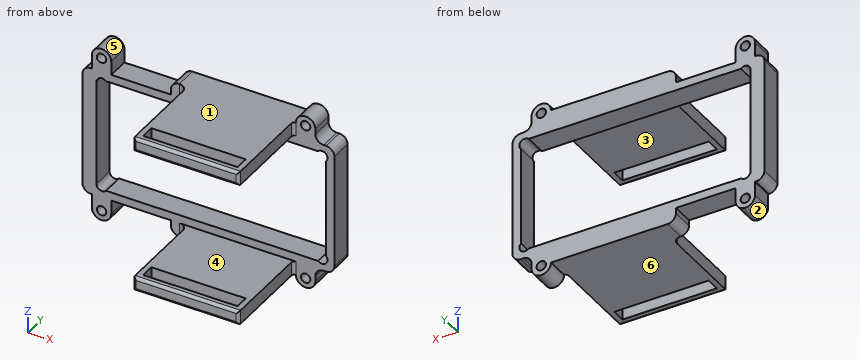
from build123d import *

# Parameters (mm, degrees)
EXTRUDE_1_DEPTH     = 23.5
EXTRUDE_START       = 8
SKETCH_2_R          = 1.7
EXTRUDE_2_DEPTH     = 8
CUT_EXTRUDE_1_REACH = 98.655
CUT_EXTRUDE_2_REACH = 79.127
CUT_EXTRUDE_3_REACH = 93.669
SKETCH_9_W          = 45
SKETCH_9_H          = 8
EXTRUDE_3_DEPTH     = 5
SKETCH_10_W         = 45
SKETCH_10_H         = 8
EXTRUDE_4_DEPTH     = 5
SKETCH_11_W         = 38
SKETCH_11_H         = 5
EXTRUDE_5_DEPTH     = 33
SKETCH_12_W         = 34
SKETCH_12_H         = 5
CUT_EXTRUDE_4_DEPTH = 5
CUT_EXTRUDE_START   = -23.5
CUT_EXTRUDE_5_DEPTH = 23.5
CUT_EXTRUDE_6_DEPTH = 67.550849919
FILLET_1_R          = 3
FILLET_2_R          = 1
FILLET_3_R          = 1


with BuildPart() as part:
    # 草图1 → 凸台-拉伸1 (new body)
    with BuildSketch(Plane(origin=(0, 0, 0), x_dir=(1, 0, 0), z_dir=(0, 1, 0))):
        with BuildLine():
            Line((-38, 23.5), (40, 23.5))
            Line((40, 23.5), (40, -23.5))
            Line((40, -23.5), (-38, -23.5))
            ThreePointArc((-38, -23.5), (-39.414213562, -22.914213562), (-40, -21.5))
            Line((-40, -21.5), (-40, 21.5))
            ThreePointArc((-40, 21.5), (-39.414213562, 22.914213562), (-38, 23.5))
        make_face()
        with BuildLine():
            Line((-34.171572875, -20.5), (36, -20.5))
            ThreePointArc((36, -20.5), (37.414213562, -19.914213562), (38, -18.5))
            Line((38, -18.5), (38, 18.5))
            ThreePointArc((38, 18.5), (37.414213562, 19.914213562), (36, 20.5))
            Line((36, 20.5), (-34.171572875, 20.5))
            ThreePointArc((-34.171572875, 20.5), (-37, 20.5), (-37, 17.671572875))
            Line((-37, 17.671572875), (-37, -17.671572875))
            ThreePointArc((-37, -17.671572875), (-37, -20.5), (-34.171572875, -20.5))
        make_face(mode=Mode.SUBTRACT)
    extrude(amount=EXTRUDE_1_DEPTH)

    # 草图2 → 凸台-拉伸2 (add)
    with BuildSketch(Plane.XZ.offset(EXTRUDE_START)):
        with BuildLine():
            Line((48.125, 23.5), (41.25, 23.5))
            Line((41.25, 23.5), (41.25, 28.5))
            ThreePointArc((41.25, 28.5), (37.75, 32), (34.25, 28.5))
            Line((34.25, 28.5), (34.25, 23.5))
            Line((34.25, 23.5), (-32.25, 23.5))
            Line((-32.25, 23.5), (-32.25, 28.5))
            ThreePointArc((-32.25, 28.5), (-35.75, 32), (-39.25, 28.5))
            Line((-39.25, 28.5), (-39.25, 23.5))
            Line((-39.25, 23.5), (-42.625, 23.5))
            Line((-42.625, 23.5), (-42.625, -23.5))
            Line((-42.625, -23.5), (-39.25, -23.5))
            Line((-39.25, -23.5), (-39.25, -28.5))
            ThreePointArc((-39.25, -28.5), (-35.75, -32), (-32.25, -28.5))
            Line((-32.25, -28.5), (-32.25, -23.5))
            Line((-32.25, -23.5), (34.25, -23.5))
            Line((34.25, -23.5), (34.25, -28.5))
            ThreePointArc((34.25, -28.5), (37.75, -32), (41.25, -28.5))
            Line((41.25, -28.5), (41.25, -23.5))
            Line((41.25, -23.5), (48.125, -23.5))
            Line((48.125, -23.5), (48.125, 23.5))
        make_face()
        with Locations(Location((37.75, 28.5, 0), (0, 0, 270))):
            Circle(SKETCH_2_R, mode=Mode.SUBTRACT)
        with Locations(Location((37.75, -28.5, 0), (0, 0, 90))):
            Circle(SKETCH_2_R, mode=Mode.SUBTRACT)
        with Locations(Location((-35.75, -28.5, 0), (0, 0, 270))):
            Circle(SKETCH_2_R, mode=Mode.SUBTRACT)
        with Locations(Location((-35.75, 28.5, 0), (0, 0, 90))):
            Circle(SKETCH_2_R, mode=Mode.SUBTRACT)
        with BuildLine():
            Line((-34.171572875, 20.5), (42.231907087, 20.5))
            ThreePointArc((42.231907087, 20.5), (45.060334211, 20.5), (45.060334211, 17.671572875))
            Line((45.060334211, 17.671572875), (45.060334211, -17.671572875))
            ThreePointArc((45.060334211, -17.671572875), (45.060334211, -20.5), (42.231907087, -20.5))
            Line((42.231907087, -20.5), (-34.171572875, -20.5))
            ThreePointArc((-34.171572875, -20.5), (-37, -20.5), (-37, -17.671572875))
            Line((-37, -17.671572875), (-37, 17.671572875))
            ThreePointArc((-37, 17.671572875), (-37, 20.5), (-34.171572875, 20.5))
        make_face(mode=Mode.SUBTRACT)
    extrude(amount=-EXTRUDE_2_DEPTH)

    # 草图4 → 切除-拉伸1 (cut, up to next)
    with BuildSketch(Plane.ZY.offset(40), mode=Mode.PRIVATE) as cut_extrude_1_sk1:
        with BuildLine():
            Line((17, 0), (-17, 0))
            ThreePointArc((-17, 0), (-19.121320344, 0.878679656), (-20, 3))
            Line((-20, 3), (-20, 17.5))
            ThreePointArc((-20, 17.5), (-19.121320344, 19.621320344), (-17, 20.5))
            Line((-17, 20.5), (17, 20.5))
            ThreePointArc((17, 20.5), (19.121320344, 19.621320344), (20, 17.5))
            Line((20, 17.5), (20, 3))
            ThreePointArc((20, 3), (19.121320344, 0.878679656), (17, 0))
        make_face()
    cut_extrude_1_tool1 = extrude(cut_extrude_1_sk1.sketch, amount=-CUT_EXTRUDE_1_REACH, mode=Mode.PRIVATE) & part.part
    add(cut_extrude_1_tool1.solids().sort_by_distance((-40, 10.25, 0))[0], mode=Mode.SUBTRACT)

    # 切除-拉伸2: up to this face of the body (flat: up to its plane)
    cut_extrude_2_end = Plane(part.part.faces().sort_by_distance((1, 8.207082452, 23.5))[0])
    # 草图5 → 切除-拉伸2 (cut, up to the picked face)
    with BuildSketch(Plane(origin=(0, 0, -23.5), x_dir=(-1, 0, 0), z_dir=(0, 0, -1)), mode=Mode.PRIVATE) as cut_extrude_2_sk1:
        with BuildLine():
            Line((-37, 11.75), (-37, 17.5))
            ThreePointArc((-37, 17.5), (-36.414213562, 18.914213562), (-35, 19.5))
            Line((-35, 19.5), (33, 19.5))
            ThreePointArc((33, 19.5), (34.414213562, 18.914213562), (35, 17.5))
            Line((35, 17.5), (35, 6))
            ThreePointArc((35, 6), (34.414213562, 4.585786438), (33, 4))
            Line((33, 4), (-35, 4))
            ThreePointArc((-35, 4), (-36.414213562, 4.585786438), (-37, 6))
            Line((-37, 6), (-37, 11.75))
        make_face()
    cut_extrude_2_tool1 = split(extrude(cut_extrude_2_sk1.sketch, amount=-CUT_EXTRUDE_2_REACH, mode=Mode.PRIVATE), bisect_by=cut_extrude_2_end, keep=Keep.BOTH, mode=Mode.PRIVATE)
    add(cut_extrude_2_tool1.solids().sort_by(Axis((1, 11.75, -23.5), (0, 0, 1)))[0], mode=Mode.SUBTRACT)

    # 草图6 → 切除-拉伸3 (cut, up to next)
    with BuildSketch(Plane(origin=(40, 0, 0), x_dir=(0, 0, -1), z_dir=(1, 0, 0)), mode=Mode.PRIVATE) as cut_extrude_3_sk1:
        with BuildLine():
            Line((21, 5), (21, 18.5))
            ThreePointArc((21, 18.5), (20.414213562, 19.914213562), (19, 20.5))
            Line((19, 20.5), (-19, 20.5))
            ThreePointArc((-19, 20.5), (-20.414213562, 19.914213562), (-21, 18.5))
            Line((-21, 18.5), (-21, 5))
            Line((-21, 5), (-21, 0))
            Line((-21, 0), (-16, 0))
            Line((-16, 0), (16, 0))
            Line((16, 0), (21, 0))
            Line((21, 0), (21, 5))
        make_face()
    cut_extrude_3_tool1 = extrude(cut_extrude_3_sk1.sketch, amount=-CUT_EXTRUDE_3_REACH, mode=Mode.PRIVATE) & part.part
    add(cut_extrude_3_tool1.solids().sort_by_distance((40, 10.230413, 0))[0], mode=Mode.SUBTRACT)

    # 草图9 → 凸台-拉伸3 (add)
    with BuildSketch(Plane.XY.offset(23.5)):
        with Locations((11.75, -4)):
            Rectangle(SKETCH_9_W, SKETCH_9_H)
    extrude(amount=EXTRUDE_3_DEPTH)

    # 草图10 → 凸台-拉伸4 (add)
    with BuildSketch(Plane(origin=(0, 0, -23.5), x_dir=(-1, 0, 0), z_dir=(0, 0, -1))):
        with Locations((-11.75, -4)):
            Rectangle(SKETCH_10_W, SKETCH_10_H)
    extrude(amount=EXTRUDE_4_DEPTH)

    # 草图11 → 凸台-拉伸5 (add)
    with BuildSketch(Plane.XZ.offset(8)):
        with Locations((14.25, 26)):
            Rectangle(SKETCH_11_W, SKETCH_11_H)
    extrude_5 = extrude(amount=EXTRUDE_5_DEPTH)

    # 草图12 → 切除-拉伸4 (cut)
    with BuildSketch(Plane(origin=(0, 0, 23.5), x_dir=(-1, 0, 0), z_dir=(0, 0, -1))):
        with Locations((-14.25, -36)):
            Rectangle(SKETCH_12_W, SKETCH_12_H)
    cut_extrude_4 = extrude(amount=-CUT_EXTRUDE_4_DEPTH, mode=Mode.SUBTRACT)

    # 镜向1: 凸台-拉伸5, 切除-拉伸4 across plane
    add(extrude_5.mirror(Plane.XY))
    add(cut_extrude_4.mirror(Plane.XY), mode=Mode.SUBTRACT)

    # 草图13 → 切除-拉伸5 (cut)
    with BuildSketch(Plane(origin=(0, 23.5, 0), x_dir=(1, 0, 0), z_dir=(0, 1, 0)).offset(CUT_EXTRUDE_START)):
        with BuildLine():
            Line((-38, 23.5), (40, 23.5))
            Line((40, 23.5), (40, -23.5))
            Line((40, -23.5), (-38, -23.5))
            ThreePointArc((-38, -23.5), (-39.414213562, -22.914213562), (-40, -21.5))
            Line((-40, -21.5), (-40, 21.5))
            ThreePointArc((-40, 21.5), (-39.414213562, 22.914213562), (-38, 23.5))
        make_face()
        with BuildLine():
            Line((38, 18.5), (38, -18.5))
            ThreePointArc((38, -18.5), (37.414213562, -19.914213562), (36, -20.5))
            Line((36, -20.5), (-34.171572875, -20.5))
            ThreePointArc((-34.171572875, -20.5), (-37, -20.5), (-37, -17.671572875))
            Line((-37, -17.671572875), (-37, 17.671572875))
            ThreePointArc((-37, 17.671572875), (-37, 20.5), (-34.171572875, 20.5))
            Line((-34.171572875, 20.5), (36, 20.5))
            ThreePointArc((36, 20.5), (37.414213562, 19.914213562), (38, 18.5))
        make_face(mode=Mode.SUBTRACT)
    extrude(amount=CUT_EXTRUDE_5_DEPTH, mode=Mode.SUBTRACT)

    # 草图14 → 切除-拉伸6 (cut, through all)
    with BuildSketch(Plane.XZ.offset(8)):
        with BuildLine():
            Line((-37.585786438, 19.085786438), (-37.585786438, -19.085786438))
            ThreePointArc((-37.585786438, -19.085786438), (-37.433545503, -18.320419573), (-37, -17.671572875))
            Line((-37, -17.671572875), (-37, 17.671572875))
            ThreePointArc((-37, 17.671572875), (-37.433545503, 18.320419573), (-37.585786438, 19.085786438))
        make_face()
    extrude(amount=-CUT_EXTRUDE_6_DEPTH, mode=Mode.SUBTRACT)

    # 圆角1
    fillet_1_edges = [part.edges().sort_by_distance(p)[0] for p in [
        (-10.75, -4, 28.5),
        (-10.75, -4, -28.5),
        (-42.625, -4, 23.5),
        (-42.625, -4, -23.5),
        (-4.75, -8, 26),
        (-4.75, -8, -26),
        (41.25, -4, 23.5),
        (41.25, -4, -23.5),
        (48.125, -4, 23.5),
        (48.125, -4, -23.5),
    ]]
    fillet(fillet_1_edges, radius=FILLET_1_R - 0.0001)  # a hair under: the kernel refuses the full size

    # 圆角2
    fillet_2_edges = [part.edges().sort_by_distance(p)[0] for p in [
        (33.25, -8, 26),
        (33.25, -8, -26),
    ]]
    fillet(fillet_2_edges, radius=FILLET_2_R)

    # 圆角3
    fillet_3_edges = [part.edges().sort_by_distance(p)[0] for p in [
        (-4.75, -41, 26),
        (14.25, -41, 23.5),
        (33.25, -41, 26),
        (14.25, -41, 28.5),
        (-4.75, -41, -26),
        (14.25, -41, -28.5),
        (33.25, -41, -26),
        (14.25, -41, -23.5),
    ]]
    fillet(fillet_3_edges, radius=FILLET_3_R)


solid = part.part
Build history of the part. All positions in model axes, mm. Face numbers are marked on the shaded views. A direction names the side the tool comes from. Coordinates: 2 decimals unless noted, no trailing zeros. Order: outer loops, then holes, each group sorted by start corner. A loop starts at its lowest first (then second) coordinate and runs counter-clockwise, first axis right, second up. Notation, with made-up numbers: (41, 72) - (60, 72) arc R24 ccw to (60, 93) - close; hole circle Ø1 at (-22, -39.5). An arc over 180 degrees is marked (long way). Write each question's results on one line, items separated by ' | '. Start each with the question number.
Item 1: Band-saw the part on B-B on y = -20.5. Write the cut outline in (x, z).
Item 2: Wall check: probe 1 along Z at (x, y) = (-26, -3.5); probe 2 along X at (y, z) = (-35.5, 26.5); probe 3 along Y at (x, z) = (26, -26). Give the ranges that are in metal, low to high. Write a range as [from, to].
Item 3: Flat gauge pins, fed straight in: pin 1 (2 mm diameter, centred on y = -10, z = 23.5, fed in from +X); pin 2 (20 mm diameter, centred on x = 11, y = -19.5, fed in from +Z); pin 3 (2.5 mm diameter, centred on x = -35.75, z = 28.5, fed in from -Y); pin 4 (5.5 mm diameter, centred on y = -36, z = 25.5, fed in from -X). Where does each tip first touch, or does it go through?
Item 4: Tool access for the marked faces 5 and 6: list every direction of +Z, -Z, +X, -X, +Y, -Y with a clear straight run to the whole face (end or side of a thin tool).
Item 5: Band-saw the part on C-C on x = 13.5. Write the cut outline in (y, z), and give its area (3 significant figures).
Item 6: Band-saw the part on D-D on y = -3. State how many separate pieces and enclosed holes the cut face has, and give its area (3 significant figures).
Item 7: Mould opens along Z. For the marked faces 1, 2, 3 and 4 say: released by +Z, released by -Z, zero draft, split by the parting line, or undercut.
Item 8: Band-saw the part on A-A on x = -29.5. Write the cut outline in (y, z), and give its area (3 significant figures).
Numbers:
1) outline: (-4.75, -28.5) - (33.25, -28.5) - (33.25, -23.5) - (-4.75, -23.5) - close; (-4.75, 23.5) - (33.25, 23.5) - (33.25, 28.5) - (-4.75, 28.5) - close
2) probe 1: [-23.5, -20.5], [20.5, 23.5] | probe 2: [-4.75, -2.75], [31.25, 33.25] | probe 3: [-41, -38.5], [-33.5, 0]
3) pin 1: x = 33.25 | pin 2: z = 28.5 | pin 3: through | pin 4: x = -4.75
4) face 5: +Z, +Y, -Y | face 6: -Z, +Y, -Y
5) outline: (-41, -27.5) arc R1 ccw to (-40, -28.5) - (-38.5, -28.5) - (-38.5, -23.5) - (-40, -23.5) arc R1 ccw to (-41, -24.5) - close; (-41, 24.5) arc R1 ccw to (-40, 23.5) - (-38.5, 23.5) - (-38.5, 28.5) - (-40, 28.5) arc R1 ccw to (-41, 27.5) - close; (-33.5, -28.5) - (0, -28.5) - (0, -20.5) - (-8, -20.5) - (-8, -23.5) - (-33.5, -23.5) - close; (-33.5, 23.5) - (-8, 23.5) - (-8, 20.5) - (0, 20.5) - (0, 28.5) - (-33.5, 28.5) - close | area: 407 mm^2
6) separate pieces: 1 | enclosed holes: 5 | area: 1,490 mm^2
7) face 1: released by +Z | face 2: released by -Z | face 3: undercut | face 4: undercut
8) outline: (-8, -23.5) - (0, -23.5) - (0, -20.5) - (-8, -20.5) - close; (-8, 20.5) - (0, 20.5) - (0, 23.5) - (-8, 23.5) - close | area: 48.0 mm^2
